```python
from build123d import *

# Parameters (mm, degrees)
SKETCH3_W          = 65.903471667
SKETCH3_H          = 42.94663955
CUT_EXTRUDE1_DEPTH = 25
SKETCH5_R          = 1.5
CUT_EXTRUDE2_DEPTH = 25


with BuildPart() as part:
    # Sketch1 → Revolve1 (revolve)
    with BuildSketch(Plane.XY):
        with BuildLine():
            Line((0, 22.4), (0, 0))
            Line((0, 0), (0, -22.4))
            ThreePointArc((0, -22.4), (-22.4, 0), (0, 22.4))
        make_face()
    revolve(axis=Axis((0, 51.787709497, 0), (0, -1, 0)))

    # Sketch3 → Cut-Extrude1 (cut, symmetric)
    with BuildSketch(Plane.XY):
        with Locations((-0.554743028, -7.473319775)):
            Rectangle(SKETCH3_W, SKETCH3_H)
    extrude(amount=CUT_EXTRUDE1_DEPTH, both=True, mode=Mode.SUBTRACT)

    # Sketch4 → Cut-Revolve1 (revolve, cut)
    with BuildSketch(Plane.XY):
        with BuildLine():
            Line((0, 0), (0, 20.9))
            ThreePointArc((0, 20.9), (-20.9, 0), (0, -20.9))
            Line((0, -20.9), (0, 0))
        make_face()
    revolve(axis=Axis((0, 39.939026177, 0), (0, -1, 0)), mode=Mode.SUBTRACT)

    # Sketch5 → Cut-Extrude2 (cut, symmetric)
    with BuildSketch(Plane(origin=(0, 0, 0), x_dir=(1, 0, 0), z_dir=(0, 1, 0))):
        Circle(SKETCH5_R)
    extrude(amount=CUT_EXTRUDE2_DEPTH, both=True, mode=Mode.SUBTRACT)


solid = part.part
```
CAD build for the part. Positions are in the model's coordinates, mm. Round coordinates to 2 decimals unless told otherwise and drop trailing zeros. Order: outer loops, then holes, each group sorted by start corner. A loop starts at its lowest first (then second) coordinate and runs counter-clockwise, first axis right, second up.
Q1. Slice it at D-D (y = 19). Write the cut outline in (x, z).
Q2. Slice it at B-B (z = 0). Write the cut outline in (x, y).
Q3. Slice it at C-C (z = -9.5). Write the cut outline in (x, y), and give its area (3 significant figures).
Q4. Wall check: L1, parallel to Z at x = 2.5, y = 15; L2, parallel to Z at x = -7.5, y = 16.75; L3, parallel to Y at x = -15, z = 3.5. Give the ranges that are in metal, low to high.
Q5. Two-plate mould, pull along X, no slides. Class faces 1 (the flat face through (-2.7, 14, -15.5)), 2 (the cylindrical face through (-0.325, 21.608, 1.464)): pulls with the +X half, pulls with the -X half, needs draft (parallel to the pull), parting line crosses it, or undercut.
Q6. Drop flat-ended pins along their axis: pin 1 (4 mm diameter, centred on x = 1.5, y = 17.5, fed in from +Z); pin 2 (3 mm diameter, centred on x = 3.5, z = 6.5, fed in from -Y); pin 3 (5 mm diameter, centred on x = 0, z = 0, fed in from -Y). Give the stop position or say it passes through.
Q7. Slice it at A-A (x = 0). Write the cut outline in (y, z).
Results below:
1. outline: circle Ø23.73 at (0, 0); hole circle Ø17.41 at (0, 0)
2. outline: (-17.49, 14) - (-15.52, 14) arc R20.9 cw to (-1.5, 20.85) - (-1.5, 22.35) arc R22.4 ccw to start; (1.5, 20.85) arc R20.9 cw to (15.52, 14) - (17.49, 14) arc R22.4 ccw to (1.5, 22.35) - close
3. outline: (-14.68, 14) - (-12.27, 14) arc R18.62 cw to (12.27, 14) - (14.68, 14) arc R20.29 ccw to start
3. area: 49.8 mm2
4. L1: z = -16.45 to -14.34, 14.34 to 16.45
4. L2: z = -12.84 to -10, 10 to 12.84
4. L3: y = 14.13 to 16.26
5. face 1: needs draft
5. face 2: undercut
6. pin 1: stops at z = 16.11
6. pin 2: stops at y = 18.92
6. pin 3: stops at y = 20.75
7. outline: (14, -17.49) arc R22.4 ccw to (22.35, -1.5) - (20.85, -1.5) arc R20.9 cw to (14, -15.52) - close; (14, 15.52) arc R20.9 cw to (20.85, 1.5) - (22.35, 1.5) arc R22.4 ccw to (14, 17.49) - close
